Input: part model. Units: mm. Frame: model coordinates. Coordinates: 2 decimals unless noted, no trailing zeros. Order: outer loops, then holes, each group sorted by start corner. A loop starts at its lowest first (then second) coordinate and runs counter-clockwise, first axis right, second up.
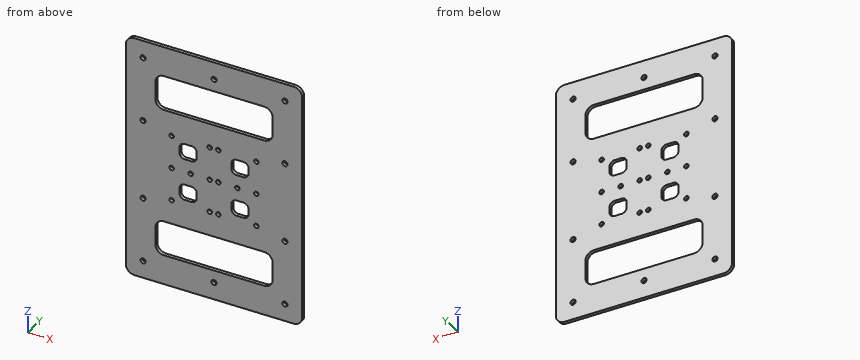
Autodesk Inventor part; units mm, degrees
ref_plane "YZ Plane" through (0, 0, 0) normal (1, 0, 0) x (0, 1, 0)
ref_plane "XZ Plane" through (0, 0, 0) normal (0, 1, 0) x (-1, 0, 0)
ref_plane "XY Plane" through (0, 0, 0) normal (0, 0, 1) x (1, 0, 0)
sketch "Sketch1" plane through (0, 0, 0) normal (0, 1, 0) x (-1, 0, 0)
  circle A0 centre (97, -135) radius 1.5
  circle A1 centre (97, -15) radius 1.5
  circle A2 centre (15, -135) radius 1.5
  circle A3 centre (15, -15) radius 1.5
  circle A4 centre (56, -135) radius 1.5
  circle A5 centre (56, -15) radius 1.5
  circle A6 centre (97, -97.9289) radius 1.5
  circle A7 centre (97, -52.0711) radius 1.5
  circle A8 centre (15, -97.9289) radius 1.5
  circle A9 centre (15, -52.0711) radius 1.5
  circle A10 centre (31.5, -94) radius 1.3
  circle A11 centre (53.5, -94) radius 1.3
  circle A12 centre (53.5, -56) radius 1.3
  circle A13 centre (31.5, -56) radius 1.3
  circle A14 centre (53.5, -75) radius 1.3
  circle A15 centre (31.5, -75) radius 1.3
  line L0 (84.9289, -42.0711) -> (27.0711, -42.0711)
  line L1 (22.0711, -37.0711) -> (22.0711, -27.0711)
  line L2 (27.0711, -22.0711) -> (84.9289, -22.0711)
  line L3 (89.9289, -27.0711) -> (89.9289, -37.0711)
  line L4 (27.0711, -127.9289) -> (84.9289, -127.9289)
  line L5 (89.9289, -122.9289) -> (89.9289, -112.9289)
  line L6 (84.9289, -107.9289) -> (27.0711, -107.9289)
  line L7 (22.0711, -112.9289) -> (22.0711, -122.9289)
  line L8 (39, -91.5) -> (43, -91.5)
  line L9 (46, -88.5) -> (46, -85.5)
  line L10 (43, -82.5) -> (39, -82.5)
  line L11 (36, -85.5) -> (36, -88.5)
  line L12 (43, -58.5) -> (39, -58.5)
  line L13 (36, -61.5) -> (36, -64.5)
  line L14 (39, -67.5) -> (43, -67.5)
  line L15 (46, -64.5) -> (46, -61.5)
  arc A16 (84.9289, -127.9289) -> (89.9289, -122.9289) centre (84.9289, -122.9289) ccw
  arc A17 (22.0711, -122.9289) -> (27.0711, -127.9289) centre (27.0711, -122.9289) ccw
  arc A18 (27.0711, -107.9289) -> (22.0711, -112.9289) centre (27.0711, -112.9289) ccw
  arc A19 (89.9289, -112.9289) -> (84.9289, -107.9289) centre (84.9289, -112.9289) ccw
  arc A20 (84.9289, -42.0711) -> (89.9289, -37.0711) centre (84.9289, -37.0711) ccw
  arc A21 (89.9289, -27.0711) -> (84.9289, -22.0711) centre (84.9289, -27.0711) ccw
  arc A22 (27.0711, -22.0711) -> (22.0711, -27.0711) centre (27.0711, -27.0711) ccw
  arc A23 (22.0711, -37.0711) -> (27.0711, -42.0711) centre (27.0711, -37.0711) ccw
  arc A24 (43, -91.5) -> (46, -88.5) centre (43, -88.5) ccw
  arc A25 (36, -88.5) -> (39, -91.5) centre (39, -88.5) ccw
  arc A26 (39, -82.5) -> (36, -85.5) centre (39, -85.5) ccw
  arc A27 (46, -85.5) -> (43, -82.5) centre (43, -85.5) ccw
  arc A28 (43, -67.5) -> (46, -64.5) centre (43, -64.5) ccw
  arc A29 (36, -64.5) -> (39, -67.5) centre (39, -64.5) ccw
  arc A30 (39, -58.5) -> (36, -61.5) centre (39, -61.5) ccw
  arc A31 (46, -61.5) -> (43, -58.5) centre (43, -61.5) ccw
  circle A32 centre (42.5, -75) radius 1.3
  circle A33 centre (80.5, -94) radius 1.3
  circle A34 centre (58.5, -94) radius 1.3
  circle A35 centre (58.5, -56) radius 1.3
  circle A36 centre (80.5, -56) radius 1.3
  circle A37 centre (58.5, -75) radius 1.3
  circle A38 centre (80.5, -75) radius 1.3
  line L16 (73, -91.5) -> (69, -91.5)
  line L17 (66, -88.5) -> (66, -85.5)
  line L18 (69, -82.5) -> (73, -82.5)
  line L19 (76, -85.5) -> (76, -88.5)
  line L20 (69, -58.5) -> (73, -58.5)
  line L21 (76, -61.5) -> (76, -64.5)
  line L22 (73, -67.5) -> (69, -67.5)
  line L23 (66, -64.5) -> (66, -61.5)
  arc A39 (66, -88.5) -> (69, -91.5) centre (69, -88.5) ccw
  arc A40 (73, -91.5) -> (76, -88.5) centre (73, -88.5) ccw
  arc A41 (76, -85.5) -> (73, -82.5) centre (73, -85.5) ccw
  arc A42 (69, -82.5) -> (66, -85.5) centre (69, -85.5) ccw
  arc A43 (66, -64.5) -> (69, -67.5) centre (69, -64.5) ccw
  arc A44 (73, -67.5) -> (76, -64.5) centre (73, -64.5) ccw
  arc A45 (76, -61.5) -> (73, -58.5) centre (73, -61.5) ccw
  arc A46 (69, -58.5) -> (66, -61.5) centre (69, -61.5) ccw
  circle A47 centre (69.5, -75) radius 1.3
  line L24 (10, -5) -> (102, -5)
  line L25 (107, -10) -> (107, -140)
  line L26 (102, -145) -> (10, -145)
  line L27 (5, -140) -> (5, -10)
  arc A48 (102, -145) -> (107, -140) centre (102, -140) ccw
  arc A49 (5, -140) -> (10, -145) centre (10, -140) ccw
  arc A50 (10, -5) -> (5, -10) centre (10, -10) ccw
  arc A51 (107, -10) -> (102, -5) centre (102, -10) ccw
  dimension "d24" = 3
  dimension "d25" = 3
  dimension "d26" = 3
  dimension "d27" = 3
  dimension "d28" = 3
  dimension "d29" = 3
  dimension "d30" = 3
  dimension "d32" = 3
  dimension "d47" = 5
  dimension "d48" = 5
  dimension "d59" = 5
  dimension "d60" = 10
  dimension "d61" = 10
  dimension "d67" = 2.6
  dimension "d71" = 140
  dimension "d72" = 102
extrude "Extrusion2" add sketch "Sketch1" along normal blind 2
properties part number "Telapak"
Item 1: Cut plane C-C on x = -83.5. Return loops of the section in (y, z), then the cut area to 3 significant figures.
Response values:
outline: (0, -145) - (2, -145) - (2, -127.93) - (0, -127.93) - close; (0, -107.93) - (2, -107.93) - (2, -42.07) - (0, -42.07) - close; (0, -22.07) - (2, -22.07) - (2, -5) - (0, -5) - close
area: 200 mm2
Item 2: Cut plane B-B on z = -15. Return loops of the section in (x, y).
Response values:
outline: (-107, 0) - (-98.5, 0) - (-98.5, 2) - (-107, 2) - close; (-95.5, 0) - (-57.5, 0) - (-57.5, 2) - (-95.5, 2) - close; (-54.5, 0) - (-16.5, 0) - (-16.5, 2) - (-54.5, 2) - close; (-13.5, 0) - (-5, 0) - (-5, 2) - (-13.5, 2) - close
Item 3: Cut plane A-A on x = -15. Return loops of the section in (y, z), then the cut area to 3 significant figures.
Response values:
outline: (0, -145) - (2, -145) - (2, -136.5) - (0, -136.5) - close; (0, -133.5) - (2, -133.5) - (2, -99.43) - (0, -99.43) - close; (0, -96.43) - (2, -96.43) - (2, -53.57) - (0, -53.57) - close; (0, -50.57) - (2, -50.57) - (2, -16.5) - (0, -16.5) - close; (0, -13.5) - (2, -13.5) - (2, -5) - (0, -5) - close
area: 256 mm2
Item 4: Ray query, probe 1 along Z at (x, y) = (-63.5, 0.35); probe 2 along Z at (x, y) = (-40.5, 1.6); probe 3 along Z at (x, y) = (-53.5, 1.1). Return the intervals inside material, ascending.
Response values:
probe 1: z = -145 to -127.93, -107.93 to -42.07, -22.07 to -5
probe 2: z = -145 to -127.93, -107.93 to -91.5, -82.5 to -67.5, -58.5 to -42.07, -22.07 to -5
probe 3: z = -145 to -127.93, -107.93 to -95.3, -92.7 to -76.3, -73.7 to -57.3, -54.7 to -42.07, -22.07 to -5
Item 5: Cut plane D-D on z = -125. Return loops of the section in (x, y).
Response values:
outline: (-107, 0) - (-89.48, 0) - (-89.48, 2) - (-107, 2) - close; (-22.52, 0) - (-5, 0) - (-5, 2) - (-22.52, 2) - close
